Verification items for the finished model (mm, model axes). A direction names the side the tool comes from. Give positions to 0.01 mm unless a question says otherwise; leave off trailing zeros. Loops run counter-clockwise (first coordinate to the right, second up) from the corner with the lowest first, then second, coordinate; pieces in that order, holes last. Notation, with made-up numbers: M 1.25,-10.75 L 43.25,-10.75 A33 cw 43.25,28.25 Z; hole C -25,71 d1. An arc over 180 degrees is marked long. Put each result on its own line as item: value. Start each with the question number.
Autodesk Inventor part; units mm, degrees
ref_plane "Work Plane1" through (0, 0, 4.572) normal (0, 0, 1) x (1, 0, 0)
ref_plane "YZ Plane" through (0, 0, 0) normal (1, 0, 0) x (0, 1, 0)
ref_plane "XZ Plane" through (0, 0, 0) normal (0, 1, 0) x (-1, 0, 0)
sketch "Sketch1" plane through (0, 0, 0) normal (0, 0, 1) x (1, 0, 0)
  arc A0 (-2.400661, 17.597517) -> (12.7, -3.175) centre (12.7, 12.7) ccw
  arc A1 (114.3, -3.175) -> (129.400661, 17.597517) centre (114.3, 12.7) ccw
  line L0 (114.3, -3.175) -> (12.7, -3.175)
  line L1 (48.399339, 174.230681) -> (-2.400661, 17.597517)
  line L2 (129.400661, 17.597517) -> (78.600661, 174.230681)
  arc A2 (78.600661, 174.230681) -> (48.399339, 174.230681) centre (63.5, 169.333164) ccw
  arc A3 (75.580529, 173.251177) -> (51.419471, 173.251177) centre (63.5, 169.333164) ccw
  arc A4 (0.619471, 16.618013) -> (12.7, 0) centre (12.7, 12.7) ccw
  arc A5 (114.3, 0) -> (126.380529, 16.618013) centre (114.3, 12.7) ccw
  line L3 (12.7, 0) -> (114.3, 0)
  line L4 (0.619471, 16.618013) -> (51.419471, 173.251177)
  line L5 (75.580529, 173.251177) -> (126.380529, 16.618013)
  line L6 (0.619471, 16.618013) -> (3.753882, 26.282436)
  line L7 (3.753882, 26.282436) -> (4.961935, 25.890635)
  circle A6 centre (4.961935, 25.890635) radius 1.27
  line L8 (51.419471, 173.251177) -> (48.285061, 163.586755)
  line L9 (48.285061, 163.586755) -> (49.493113, 163.194953)
  circle A7 centre (49.493113, 163.194953) radius 1.27
  circle A8 centre (27.227524, 94.542794) radius 1.27
  line L10 (75.580529, 173.251177) -> (78.714939, 163.586755)
  line L11 (78.714939, 163.586755) -> (77.506886, 163.194953)
  circle A9 centre (77.506886, 163.194953) radius 1.27
  line L12 (126.380529, 16.618013) -> (123.246118, 26.282436)
  line L13 (123.246118, 26.282436) -> (122.038065, 25.890635)
  circle A10 centre (122.038065, 25.890635) radius 1.27
  circle A11 centre (99.772476, 94.542794) radius 1.27
  line L14 (63.5, 0) -> (63.5, 1.27) construction
  line L15 (63.5, 1.27) -> (76.2, 1.27) construction
  line L16 (63.5, 1.27) -> (50.8, 1.27) construction
  circle A12 centre (50.8, 1.27) radius 1.27
  circle A13 centre (76.2, 1.27) radius 1.27
  point P0 (0, 0)
  point P1 (0, 0)
  dimension "d50" = 2.54
  dimension "d53" = 2.54
  dimension "d39" = 31.75
  dimension "d40" = 31.75
  dimension "d41" = 25.4
  dimension "d42" = 25.4
  dimension "d43" = 25.4
  dimension "d44" = 10.16
  dimension "d45" = 10.16
  dimension "d46" = 1.27
  dimension "d47" = 1.27
  dimension "d48" = 10.16
  dimension "d49" = 10.16
  dimension "d51" = 2.54
  dimension "d52" = 2.54
  dimension "d91" = 12.7
  dimension "d92" = 12.7
ref_plane "Work Plane1" through (0, 0, 4.572) normal (0, 0, 1) x (1, 0, 0)
sketch "Sketch2" plane through (0, 0, 4.572) normal (0, 0, 1) x (1, 0, 0)
  line L0 (12.7, -3.175) -> (114.3, -3.175)
  line L1 (34.171935, 12.065) -> (34.171935, 67.945) construction
  line L2 (34.171935, 67.945) -> (86.241935, 67.945) construction
  line L3 (86.241935, 67.945) -> (86.241935, 12.065) construction
  line L4 (86.241935, 12.065) -> (34.171935, 12.065) construction
  line L5 (34.171935, 12.065) -> (86.241935, 67.945) construction
  line L6 (34.171935, 67.945) -> (86.241935, 12.065) construction
  circle A0 centre (34.171935, 67.945) radius 1.27
  circle A1 centre (34.171935, 12.065) radius 1.27
  circle A2 centre (86.241935, 12.065) radius 1.27
  circle A3 centre (86.241935, 67.945) radius 1.27
  circle A4 centre (4.961935, 25.890635) radius 1.27
  arc A5 (78.600661, 174.230681) -> (48.399339, 174.230681) centre (63.5, 169.333164) ccw
  point P0 (0, 0)
  point P1 (60.206935, 40.005)
  dimension "d71" = 55.88
  dimension "d73" = 52.07
  dimension "d74" = 2.54
  dimension "d75" = 2.54
  dimension "d76" = 2.54
  dimension "d77" = 2.54
  dimension "d80" = 52.07
  dimension "d81" = 15.24
  dimension "d82" = 29.21
sketch "Sketch1 outline for Extrusion8" plane through (0, 0, 0) normal (0, 0, 1) x (1, 0, 0)
  arc A0 (78.600661, 174.230681) -> (48.399339, 174.230681) centre (63.5, 169.333164) ccw
  line L0 (129.400661, 17.597517) -> (78.600661, 174.230681)
  line L1 (48.399339, 174.230681) -> (-2.400661, 17.597517)
  arc A1 (114.3, -3.175) -> (129.400661, 17.597517) centre (114.3, 12.7) ccw
  arc A2 (-2.400661, 17.597517) -> (12.7, -3.175) centre (12.7, 12.7) ccw
  line L2 (12.7, -3.175) -> (114.3, -3.175)
  circle A3 centre (4.961935, 25.890635) radius 1.27
  circle A4 centre (50.8, 1.27) radius 1.27
  circle A5 centre (76.2, 1.27) radius 1.27
  circle A6 centre (122.038065, 25.890635) radius 1.27
  circle A7 centre (27.227524, 94.542794) radius 1.27
  circle A8 centre (49.493113, 163.194953) radius 1.27
  circle A9 centre (99.772476, 94.542794) radius 1.27
  circle A10 centre (77.506886, 163.194953) radius 1.27
extrude "Extrusion8" add sketch "Sketch1 outline for Extrusion8" along normal blind 4.572
sketch "Sketch3" plane through (0, 0, 4.572) normal (0, 0, 1) x (1, 0, 0)
  circle A0 centre (76.2, 1.27) radius 1.27
  line L0 (76.2, 1.27) -> (117.405446, 1.27)
  line L1 (117.405446, 1.27) -> (117.405446, 3.556)
  line L2 (76.2, 3.556) -> (76.2, 1.27)
  line L3 (107.52753, 3.556) -> (107.52753, 9.906)
  line L4 (107.52753, 9.906) -> (94.82753, 9.906)
  line L5 (94.82753, 9.906) -> (94.82753, 3.556)
  circle A1 centre (101.17753, 25.503714) radius 2.794
  line L6 (12.7, -3.175) -> (114.3, -3.175)
  line L7 (63.5, -3.175) -> (63.5, 31.793571) construction
  line L8 (101.17753, 8.001) -> (63.5, 8.001) construction
  line L9 (107.52753, 3.556) -> (107.52753, 1.27)
  line L10 (107.52753, 1.27) -> (94.82753, 1.27)
  line L11 (94.82753, 1.27) -> (94.82753, 3.556)
  line L12 (117.405446, 3.556) -> (107.52753, 3.556)
  line L13 (94.82753, 3.556) -> (76.2, 3.556)
  point P0 (0, 0)
  dimension "d97" = 2.286
  dimension "d98" = 12.7
  dimension "d99" = 6.35
  dimension "d106" = 5.588
  dimension "d109" = 37.67753
extrude "Extrusion10" cut sketch "Sketch3" against normal blind 25.4 contours L11 L5 L4 L3 L9 L0 | A1
fillet "Fillet1" radius 0.635 1 edges at (94.8275, 9.906, 2.286)
fillet "Fillet2" radius 0.635 1 edges at (107.5275, 9.906, 2.286)
extrude "Extrusion11" cut sketch "Sketch2" against normal blind 25.4 contours A0 | A1 | A2 | A3
fillet "Fillet5" radius 0.635 1 edges at (94.8275, 1.27, 2.286)
fillet "Fillet6" radius 0.635 1 edges at (107.5275, 1.27, 2.286)
properties part number "Nathan_LED_Speaker_Back"
Q1. Set-up check for faces 4 (the face through (23.355, 97.011, 2.254)), 5 (the face through (101, 9.906, 2)): record each of +Z, -Z, +X, -X, +Y, -Y from which the full face is reachable in a straight line by a thin tool's end or side.
Q2. Cross-section at C-C, the plane y = 107.5. Record the boundary of the cut face in (x, z), then the cut area to 3 significant figures.
Q3. Cross-section at B-B, the plane x = 41. Record the boundary of the cut face in (y, z) (3 decimals).
Q4. Scan lines: L1, parallel to X at y = 11, z = 3.7; L2, parallel to Y at x = 74.5, z = 0.9 (3 decimals); L3, parallel to X at y = 159, z = 2.6. Record each from-to range of solid material in increasing order.
Q5. Cross-section at A-A, the plane z = 3.75. State how many separate pieces and enclosed holes the cut face has, then the cut area to 3 significant figures.
Q6. Release check for a two-part mould opening along Y. For faces 1 (the face through (63, -3.175, 2)), 2 (the face through (94.828, 6, 2)), 3 (the face through (104.356, 94.818, 2.254)) record: pulls with the +Y half, pulls with the -Y half, needs draft (parallel to the pull), parting line crosses it, or undercut.
Q7. Go/stop test with flat-tipped pins: pin 1 (2 mm diameter, centred on y = 145, z = 3.5, fed in from -X); pin 2 (1.5 mm diameter, centred on y = 140.5, z = 2, fed in from -X). Record where each tip stops, or that it passes through.
Ans:
1. face 4: +Z, -Z, -X, +Y
1. face 5: +Z, -Z
2. outline: M 26.76,0 L 100.24,0 L 100.24,4.57 L 26.76,4.57 Z
2. area: 336 mm^2
3. outline: M -3.175,0 L 151.416,0 L 151.416,4.572 L -3.175,4.572 Z
4. L1: x = -3.08 to 33.48, 34.86 to 85.55, 86.93 to 130.08
4. L2: y = -3.175 to 180.779
4. L3: x = 43.46 to 83.54
5. separate pieces: 1
5. enclosed holes: 14
5. area: 15,400 mm^2
6. face 1: pulls with the -Y half
6. face 2: undercut
6. face 3: pulls with the +Y half
7. pin 1: stops at x = 38.59
7. pin 2: stops at x = 37.22
